Autodesk Inventor part; units mm, degrees
ref_plane "YZ Plane" through (0, 0, 0) normal (1, 0, 0) x (0, 1, 0)
ref_plane "XZ Plane" through (0, 0, 0) normal (0, 1, 0) x (-1, 0, 0)
ref_plane "XY Plane" through (0, 0, 0) normal (0, 0, 1) x (1, 0, 0)
sketch "Эскиз1" plane through (0, 0, 0) normal (0, 1, 0) x (-1, 0, 0)
  line L0 (0, 0) -> (0, -5)
  line L1 (0, -5) -> (12, -5)
  line L2 (14, 0) -> (14, -4.75)
  line L3 (14, -4.75) -> (13, -4.75)
  line L4 (12, -4.75) -> (12, -5)
  line L5 (14, 0) -> (14, -8)
  line L6 (14, -8) -> (19, -8)
  line L7 (19, 0) -> (64, 0)
  line L8 (64, -5) -> (64, -5.5)
  line L9 (64, -5.5) -> (19, -8)
  line L10 (64, -5.5) -> (64, -5)
  line L11 (64, -5) -> (74, -5)
  line L12 (74, -5) -> (74, 0)
  line L13 (74, 0) -> (0, 0)
  line L14 (14, -4.75) -> (14, -5.75)
  line L15 (14, -5.75) -> (13, -5.75)
  arc A0 (14, -5.75) -> (13, -4.75) centre (13, -5.75) ccw
  line L16 (13, -4.75) -> (12, -5)
  dimension "d0" = 5
  dimension "d1" = 12
  dimension "d3" = 2
  dimension "d5" = 5
  dimension "d6" = 45
  dimension "d7" = 5.5
  dimension "d8" = 0.5
  dimension "d9" = 10
  dimension "d25" = 1
revolve "Вращение1" add sketch "Эскиз1" angle 360 about axis through (-74, 0, 0) along (1, 0, 0)
thread "Резьба1"
sketch "Эскиз2" plane through (0, 0, 0) normal (0, 1, 0) x (-1, 0, 0)
  line L0 (14, 5.0083) -> (6, 5)
  line L1 (12, 5) -> (0, 5)
  line L2 (6, 5) -> (9.0413, -6.3501)
  line L3 (6, 5) -> (17.7505, 5) construction
  line L4 (9.0413, -6.3501) -> (10.4902, -5.9619)
  line L5 (10.4902, -5.9619) -> (6.6566, 8.345)
  line L6 (6.6566, 8.345) -> (5.2077, 7.9567)
  line L7 (5.2077, 7.9567) -> (9.0413, -6.3501)
  point P0 (0, 0)
  point P1 (7.5525, 5.0016)
  dimension "d13" = 8
  dimension "d14" = 75
  dimension "d15" = 1.5
  dimension "d16" = 1.5
revolve "Вращение2" cut sketch "Эскиз2" angle 360 about axis through (-5.2077, 0, 7.9567) along (-0.2588, 0, -0.9659)
chamfer "Фаска1" distance 1 angle 45 1 edges at (0, 0, 5)
chamfer "Фаска2" distance 1.6 angle 45 1 edges at (-74, 0, 5)
properties part number "Рукоятка-8"
Geometry: final body of the model. Coordinates: model frame, mm. A direction names the side the tool comes from. Coordinates: 2 decimals unless noted, no trailing zeros. Order: outer loops, then holes, each group sorted by start corner. A loop starts at its lowest first (then second) coordinate and runs counter-clockwise, first axis right, second up.
1) Section C-C (x = -69). Return loops of the section in (y, z), then the cut area to 3 significant figures.
Result sheet:
outline: circle Ø10 at (0, 0)
area: 78.5 mm2
2) First-contact query: P1, Ø1, axis at x = -18, y = -4, coming from the -Z side; P2, Ø2, axis at x = -66, z = -2.5, coming from the +Y side; P3, Ø6, axis at x = -49, y = -5, coming from the -Z side. Flat tips, straight axial feed; report the tip coordinate or a pass-through.
Result sheet:
P1: stops at z = -7.19
P2: stops at y = 4.77
P3: stops at z = -6.02
3) Section B-B (x = -15.5). Return loops of the section in (y, z), then the cut area to 3 significant figures.
Result sheet:
outline: circle Ø16 at (0, 0)
area: 201 mm2
4) Draft query along X for faces 1 (the flat face through (-14, -3.4, -5.2)), 2 (the cylindrical face through (-7.131, -1.487, 0.025)), 3 (the cylindrical face through (-16.54, 7.81, 1.73)). Return one class per face: released by +X, released by -X, zero draft, split by the parting line, or undercut.
Result sheet:
face 1: released by +X
face 2: undercut
face 3: zero draft
5) Section A-A (y = 0). Return loops of the section in (x, z), then the cut area to 3 significant figures.
Result sheet:
outline: (-74, -3.4) - (-72.4, -5) - (-64, -5) - (-64, -5.5) - (-19, -8) - (-14, -8) - (-14, -5.75) arc R1 cw to (-13, -4.75) - (-12, -5) - (-10.23, -5) - (-7.55, 5) - (-12, 5) - (-13, 4.75) arc R1 cw to (-14, 5.75) - (-14, 8) - (-19, 8) - (-64, 5.5) - (-64, 5) - (-72.4, 5) - (-74, 3.4) - close; (-7.13, -5) - (-1, -5) - (0, -4) - (0, 4) - (-1, 5) - (-4.45, 5) - close
area: 893 mm2
6) Set-up query: faces 4 (the cylindrical face through (-6.58, -1.5, -4.77)), 5 (the flat face through (-74, 0, 0)), 6 (the flat face through (-64, -4.9, -1.6)). Return all of +Z, -Z, +X, -X, +Y, -Y with unobstructed straight access to the full face (end or side cutting, diameter ignored); none if empty.
Result sheet:
face 4: +X
face 5: +Z, -Z, -X, +Y, -Y
face 6: -X
7) Ray query, probe 1 along X at (y, z) = (0, -2.25); probe 2 along Z at (x, y) = (-5, -3); probe 3 along Z at (x, y) = (-41, -1.5). Return the intervals inside material, ascending.
Result sheet:
probe 1: x = -74 to -9.5, -6.39 to 0
probe 2: z = -4 to 4
probe 3: z = -6.61 to 6.61
